The listing builds one solid part. Answer for the finished solid, in the listing's coordinates (mm). Face numbers are marked on the shaded views. A direction names the side the tool comes from. Give positions to 0.01 mm unless a question says otherwise; leave off trailing zeros. Order: outer loops, then holes, each group sorted by start corner. A loop starts at its lowest first (then second) coordinate and runs counter-clockwise, first axis right, second up. Notation, with made-up numbers: (-25, -10) - (-4, -10) arc R20 ccw to (-4, 15) - close; hole circle Ø9 at (31, 41). An arc over 180 degrees is marked (long way). Answer in a Markdown table with one row per item. Add a question column.
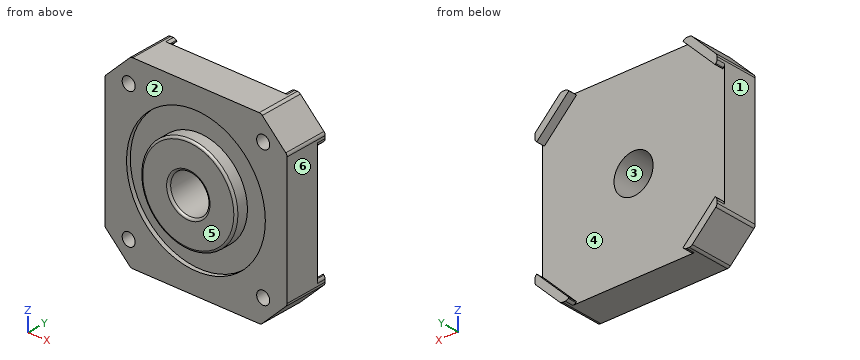
Autodesk Inventor part; units mm, degrees
ref_plane "YZ Plane" through (0, 0, 0) normal (1, 0, 0) x (0, 1, 0)
ref_plane "XZ Plane" through (0, 0, 0) normal (0, 1, 0) x (-1, 0, 0)
ref_plane "XY Plane" through (0, 0, 0) normal (0, 0, 1) x (1, 0, 0)
sketch "Sketch1" plane through (0, 0, 0) normal (0, 1, 0) x (-1, 0, 0)
  line L0 (-21, -21) -> (21, -21)
  line L1 (21, -21) -> (21, 21)
  line L2 (21, 21) -> (-21, 21)
  line L3 (-21, 21) -> (-21, -21)
  line L4 (-21, -21) -> (21, 21) construction
  line L5 (21, -21) -> (-21, 21) construction
  point P0 (0, 0)
  dimension "d0" = 42
  dimension "d1" = 42
extrude "Extrusion1" add sketch "Sketch1" along normal blind 8
sketch "Sketch2" plane through (0, 0, 0) normal (0, -1, 0) x (1, 0, 0)
  point P0 (0, 0)
chamfer "Chamfer1" distance 6 angle 45 4 edges at (-21, 4, 21) (21, 4, 21) (21, 4, -21) (-21, 4, -21)
sketch "Sketch3" plane through (0, 8, 0) normal (0, 1, 0) x (1, 0, 0)
  line L0 (-21, 15) -> (-15, 21)
  line L1 (-21, 15) -> (-21, -15)
  line L2 (-15, -21) -> (-21, -15)
  line L3 (-15, -21) -> (15, -21)
  line L4 (21, -15) -> (15, -21)
  line L5 (21, -15) -> (21, 15)
  line L6 (15, 21) -> (21, 15)
  line L7 (15, 21) -> (-15, 21)
  line L8 (-19.6609, -14.0495) -> (-13.6609, -20.0495)
  line L9 (-15, -21) -> (-21, -15)
  line L10 (-21, -15) -> (-19.8552, -13.8552)
  line L11 (-19.8552, -13.8552) -> (-19.6609, -14.0495)
  line L12 (-15, -21) -> (-13.8552, -19.8552)
  line L13 (-13.6609, -20.0495) -> (-13.1481, -20.5623)
  line L14 (-13.1481, -20.5623) -> (-13.5858, -21)
  line L15 (-19.8552, -13.8552) -> (-20.5623, -13.1481)
  line L16 (-20.5623, -13.1481) -> (-21, -13.5858)
  point P0 (0, 0)
  dimension "d11" = 1
  dimension "d12" = 1
extrude "Extrusion2" add sketch "Sketch3" along normal blind 2 contours L16 L15 L10 L1 | L10 L11 L8 L12 L2 | L12 L8 L13 L14 L3
mirror "Mirror1" about plane through (0, 0, 0) normal (0, 0, 1) of "Extrusion2"
mirror "Mirror2" about plane through (0, 0, 0) normal (1, 0, 0) of "Extrusion2", "Mirror1"
fillet "Fillet2" radius 1 8 edges at (15, 5, -21) (21, 5, -15) (21, 5, 15) (15, 5, 21) (-15, 5, 21) (-21, 5, 15) (-21, 5, -15) (-15, 5, -21)
fillet "Fillet3" radius 1 8 edges at (-21, 9, 13.5858) (-13.5858, 9, 21) (13.5858, 9, 21) (21, 9, 13.5858) (21, 9, -13.5858) (13.5858, 9, -21) (-13.5858, 9, -21) (-21, 9, -13.5858)
sketch "Sketch4" plane through (0, 0, 0) normal (0, -1, 0) x (1, 0, 0)
  circle A0 centre (0, 0) radius 16
  circle A1 centre (0, 0) radius 11
  dimension "d14" = 32
  dimension "d15" = 22
extrude "Extrusion3" cut sketch "Sketch4" against normal blind 1
sketch "Sketch5" plane through (0, 0, 0) normal (0, -1, 0) x (1, 0, 0)
  circle A0 centre (0, 0) radius 11
extrude "Extrusion4" add sketch "Sketch5" along normal blind 2
sketch "Sketch6" plane through (0, -2, 0) normal (0, -1, 0) x (1, 0, 0)
  circle A0 centre (0, 0) radius 4.5
  dimension "d20" = 9
extrude "Extrusion5" cut sketch "Sketch6" against normal up to surface (10 mm away)
sketch "Sketch7" plane through (0, 0, 0) normal (0, -1, 0) x (1, 0, 0)
  point P0 (0, 0)
sketch "Sketch8" plane through (0, 0, 0) normal (0, -1, 0) x (1, 0, 0)
  circle A0 centre (-15.5, -15.5) radius 1.5
  line L0 (14.5858, -21) -> (-14.5858, -21)
  line L1 (-21, -14.5858) -> (-21, 14.5858)
  point P0 (0, 0)
  dimension "d23" = 3
  dimension "d24" = 5.5
  dimension "d25" = 5.5
extrude "Extrusion6" cut sketch "Sketch8" against normal blind 5
mirror "Mirror3" about plane through (0, 0, 0) normal (0, 0, 1) of "Extrusion6"
mirror "Mirror4" about plane through (0, 0, 0) normal (1, 0, 0) of "Extrusion6", "Mirror3"
fillet "Fillet4" radius 0.5 1 edges at (-11, -2, 0)
fillet "Fillet5" radius 0.5 1 edges at (-4.5, -2, 0)
equation "\"d12\" = d11"
equation "\"d25\" = d24"
(1) Find section D-D, the plane y = 6.75. Write down the section's boundary in (x, z).
(2) Find section B-B, the plane z = 0. Write down the section's boundary in (x, y).
(3) For the marked faces 1 and 2, determine the directions among +Z, -Z, +X, -X, +Y, -Y from which every point of the face is accessible in a straight line to the end or side of a thin tool.
(4) Each of these flat-tipped pins is pushed along its axis until it touches: P1, Ø4, axis at x = 15.5, z = 15.5, coming from the -Y side; P2, Ø12, axis at x = 14.5, z = -3.5, coming from the +Y side; P3, Ø2.5, axis at x = -15.5, z = 15.5, coming from the -Y side. Where does it stop, or does it pass through?
(5) Find section A-A, the plane y = 2.5. Write down the section's boundary in (x, z).
(6) Straight lines are drawn through the part: line 1 (Z direction, x = 0, y = 3.5); line 2 (Z direction, x = -15.5, y = 3.75); line 3 (Z direction, x = -9, y = 0.25). For each, find the intervals that lie inside material, in ascending order.
(7) The mould has two halves that part along X. Classify the marked faces 3, 4, 5 and 6: +X half, -X half, draft (parallel to the pull), parting line (faces both ways), or undercut.
(8) Find section C-C, the plane x = 0. Write down the section's boundary in (y, z).
Answer key:
| question | item | result |
|---|---|---|
| 1 | outline | (-21, -14.59) arc R1 ccw to (-20.71, -15.29) - (-15.29, -20.71) arc R1 ccw to (-14.59, -21) - (14.59, -21) arc R1 ccw to (15.29, -20.71) - (20.71, -15.29) arc R1 ccw to (21, -14.59) - (21, 14.59) arc R1 ccw to (20.71, 15.29) - (15.29, 20.71) arc R1 ccw to (14.59, 21) - (-14.59, 21) arc R1 ccw to (-15.29, 20.71) - (-20.71, 15.29) arc R1 ccw to (-21, 14.59) - close; hole circle Ø9 at (0, 0) |
| 2 | outline | (-21, 0) - (-16, 0) - (-16, 1) - (-11, 1) - (-11, -1.5) arc R0.5 ccw to (-10.5, -2) - (-5, -2) arc R0.5 ccw to (-4.5, -1.5) - (-4.5, 8) - (-21, 8) - close; (4.5, -1.5) arc R0.5 ccw to (5, -2) - (10.5, -2) arc R0.5 ccw to (11, -1.5) - (11, 1) - (16, 1) - (16, 0) - (21, 0) - (21, 8) - (4.5, 8) - close |
| 3 | face 1 | +Z, -Z, -X, +Y, -Y |
| 3 | face 2 | -Y |
| 4 | P1 | y = 0 |
| 4 | P2 | y = 8 |
| 4 | P3 | y = 5 |
| 5 | outline | (-21, -14.59) arc R1 ccw to (-20.71, -15.29) - (-15.29, -20.71) arc R1 ccw to (-14.59, -21) - (14.59, -21) arc R1 ccw to (15.29, -20.71) - (20.71, -15.29) arc R1 ccw to (21, -14.59) - (21, 14.59) arc R1 ccw to (20.71, 15.29) - (15.29, 20.71) arc R1 ccw to (14.59, 21) - (-14.59, 21) arc R1 ccw to (-15.29, 20.71) - (-20.71, 15.29) arc R1 ccw to (-21, 14.59) - close; hole circle Ø3 at (-15.5, -15.5); hole circle Ø3 at (-15.5, 15.5); hole circle Ø9 at (0, 0); hole circle Ø3 at (15.5, -15.5); hole circle Ø3 at (15.5, 15.5) |
| 6 | line 1 | -21 to -4.5, 4.5 to 21 |
| 6 | line 2 | -20.5 to -17, -14 to 14, 17 to 20.5 |
| 6 | line 3 | -21 to -13.23, -6.32 to 6.32, 13.23 to 21 |
| 7 | face 3 | undercut |
| 7 | face 4 | undercut |
| 7 | face 5 | draft |
| 7 | face 6 | +X half |
| 8 | outline | (-2, -10.5) arc R0.5 ccw to (-1.5, -11) - (1, -11) - (1, -16) - (0, -16) - (0, -21) - (8, -21) - (8, -4.5) - (-1.5, -4.5) arc R0.5 ccw to (-2, -5) - close; (-2, 5) arc R0.5 ccw to (-1.5, 4.5) - (8, 4.5) - (8, 21) - (0, 21) - (0, 16) - (1, 16) - (1, 11) - (-1.5, 11) arc R0.5 ccw to (-2, 10.5) - close |
